Autodesk Fusion 360 part; units mm, degrees
sketch "Sketch1" plane through (0, 0, 0) normal (0, 0, 1) x (1, 0, 0)
  circle A0 centre (0, 0) radius 21.463
  dimension "d1" = 42.926
extrude "Extrude1" add sketch "Sketch1" along normal blind 5
sketch "Sketch2" plane through (0, 0, 5) normal (0, 0, 1) x (-1, 0, 0)
  circle A0 centre (0, 0) radius 21.463
  circle A1 centre (0, 0) radius 3.175
  dimension "d4" = 6.35
extrude "Extrude2" add sketch "Sketch2" along normal blind 9.4996 contours A1
thread "Thread1" thread offset 0 thread length 10.0076
move_face "OffsetFaces1" offset 1.651 1 faces at (1.0387, 4.551, 0)
equation "d5 = -0.385 in + 0.709 in + 0.05 in"
equation "d9 = 0.262 in - 0.197 in"
Input: part model. Units: mm. Frame: model coordinates. A direction names the side the tool comes from. Coordinates: 2 decimals unless noted, no trailing zeros. Loops run counter-clockwise (first coordinate to the right, second up) from the corner with the lowest first, then second, coordinate; pieces in that order, holes last. Notation, with made-up numbers: (-17.75, 29.25) -> (9.25, 29.25) arc R19 ccw to (9.25, 44.25) -> close; hole circle Ø7 at (21.5, 9.5). An arc over 180 degrees is marked (long way). Write each question's results on one line, items separated by ' | '. Start each with the question number.
Q1. Section A-A, the plane x = 0. Return the cut outline in (y, z) (3 decimals), plus the area to 3 significant figures.
Q2. Pin query (flat end, axial travel): pin 1 (6 mm diameter, centred on x = -8.5, y = 16.5, fed in from +Z); pin 2 (4 mm diameter, centred on x = 16.5, z = 0.5, fed in from -Y). Return the tip coordinate at first contact, or that it passes through.
Q3. Section C-C, the plane z = 8.25. Return the cut outline in (x, y) (3 decimals).
Q4. Ray query, line 1 (Z direction, x = 8, y = -13); line 2 (X direction, y = -8.5, z = -0.25); line 3 (Y direction, x = 11, z = 1.5). Return the intervals inside material, ascending. Write a range as from..to.
Q5. Reachability of faces 1 (the cylindrical face through (20.47, -6.45, 1.63)), 2 (the cylindrical face through (0.69, -3.1, 9.68)) from +Z, -Z, +X, -X, +Y, -Y: full face, straight path, thin tool, end or side. Return the list, or none.
Q6. Section D-D, the plane y = -9.5. Return the cut outline in (x, z), plus the area to 3 significant figures.
Found:
1) outline: (-21.463, -1.651) -> (21.463, -1.651) -> (21.463, 5) -> (3.175, 5) -> (3.175, 14.5) -> (-3.175, 14.5) -> (-3.175, 5) -> (-21.463, 5) -> close | area: 346 mm2
2) pin 1: z = 5 | pin 2: y = -15.82
3) outline: circle Ø6.35 at (0, 0)
4) line 1: -1.65..5 | line 2: -19.71..19.71 | line 3: -18.43..18.43
5) face 1: +Z, -Z | face 2: +Z
6) outline: (-19.25, -1.65) -> (19.25, -1.65) -> (19.25, 5) -> (-19.25, 5) -> close | area: 256 mm2
